Answer from the drawing. Dimensions are ordinates in mm from the lowest x, y and z of the part. Coordinates: 2 decimals unless noted, no trailing zeros. Write each loop counter-clockwise with the first axis right and the second up, starting at its lowest first coordinate (ties: lowest second). Pieces come first, ordered by that corner, then holes.
(1) The part is cut by section D-D, the plane x = 22.75. Determine the outline of the cut face in (y, z), and give its area (3 significant figures).
(2) The part is cut by section B-B, the plane x = 14.85. Determine the outline of the cut face in (y, z), and give its area (3 significant figures).
(3) The part is cut by section A-A, the plane z = 32.35. Determine the outline of the cut face in (x, y) (3 decimals), and give its area (3 significant figures).
(4) The part is cut by section C-C, the plane z = 12.5. Determine the outline of the cut face in (x, y), and give its area (3 significant figures).
(5) Straight lines are drawn through the part: line 1 along X through (y, z) = (0.9, 32.35) (3 decimals); line 2 along Z through (x, y) = (14.75, 1.15); line 3 along X through (y, z) = (1.3, 14.85). For each, find the intervals that lie inside material, in ascending order.
(6) Given pin 1 (1 mm diameter, centred on y = 1.5, z = 14, fed in from +X), flat-ended and moving along its own axis, determine where the tip first touches the part or whether it passes through.
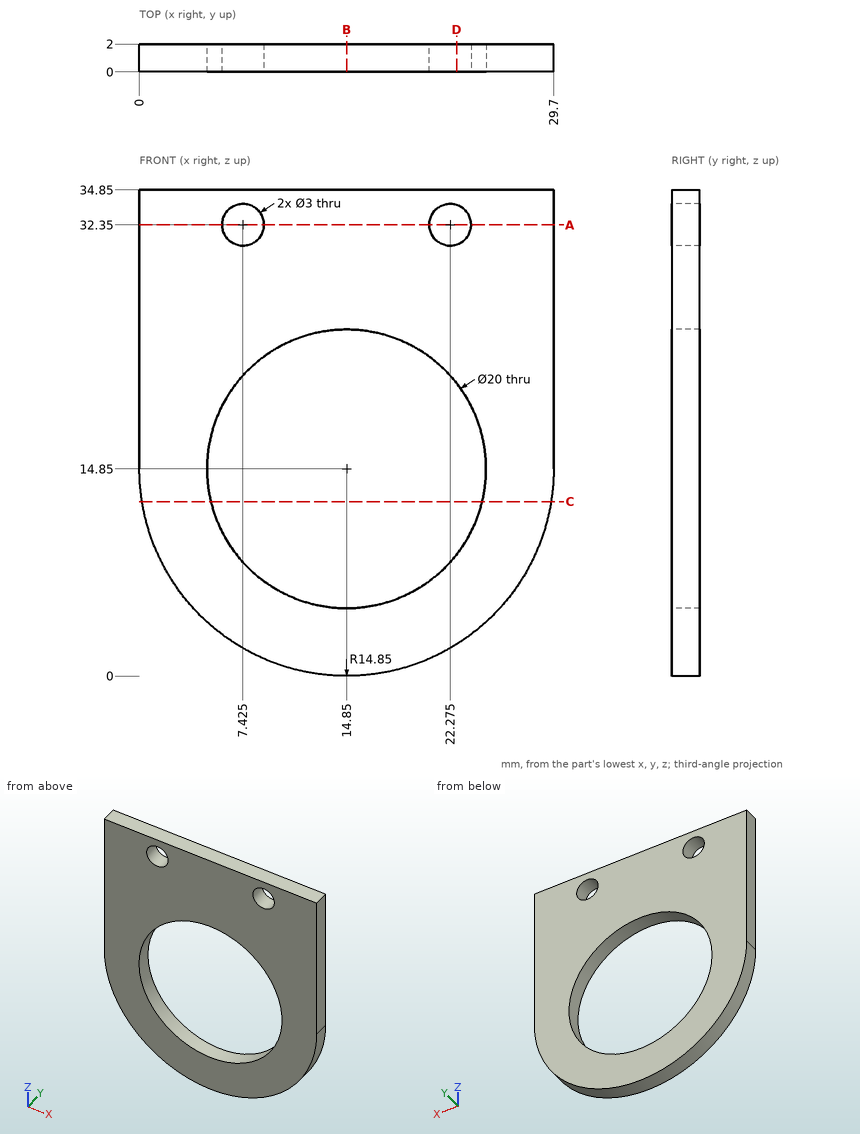
Computed:
1. outline: (0, 2.28) - (2, 2.28) - (2, 8.72) - (0, 8.72) - close; (0, 20.98) - (2, 20.98) - (2, 30.93) - (0, 30.93) - close; (0, 33.77) - (2, 33.77) - (2, 34.85) - (0, 34.85) - close
1. area: 34.9 mm2
2. outline: (0, 0) - (2, 0) - (2, 4.85) - (0, 4.85) - close; (0, 24.85) - (2, 24.85) - (2, 34.85) - (0, 34.85) - close
2. area: 29.7 mm2
3. outline: (0, 0) - (5.925, 0) - (5.925, 2) - (0, 2) - close; (8.925, 0) - (20.775, 0) - (20.775, 2) - (8.925, 2) - close; (23.775, 0) - (29.7, 0) - (29.7, 2) - (23.775, 2) - close
3. area: 47.4 mm2
4. outline: (0.19, 0) - (5.13, 0) - (5.13, 2) - (0.19, 2) - close; (24.57, 0) - (29.51, 0) - (29.51, 2) - (24.57, 2) - close
4. area: 19.8 mm2
5. line 1: x = 0 to 5.925, 8.925 to 20.775, 23.775 to 29.7
5. line 2: z = 0 to 4.85, 24.85 to 34.85
5. line 3: x = 0 to 4.85, 24.85 to 29.7
6. pin 1: stops at x = 29.7
